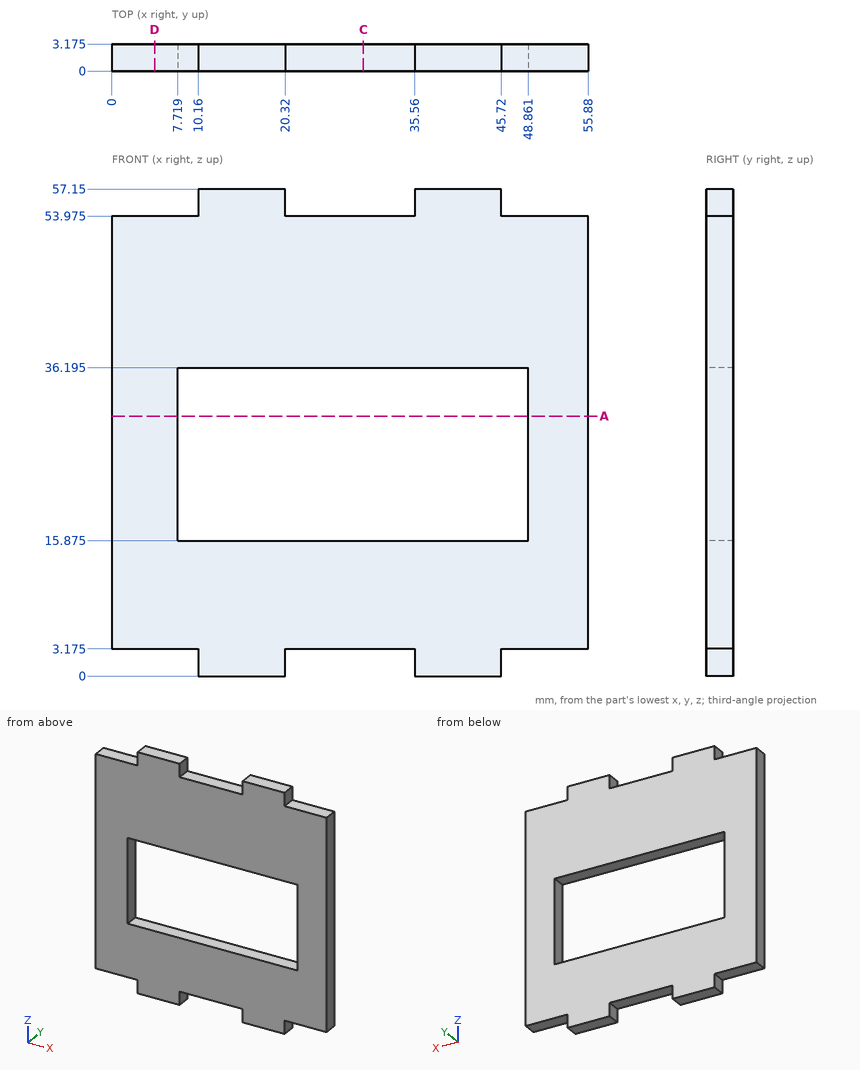
Drawing for the job (mm, zero at the part's lowest x, y, z). Round coordinates to 2 decimals unless told otherwise and drop trailing zeros. Order: outer loops, then holes, each group sorted by start corner. A loop starts at its lowest first (then second) coordinate and runs counter-clockwise, first axis right, second up.
Item 1: Saw through at C-C on x = 29.5. Write the cut outline in (y, z) (1 decimal).
Item 2: Saw through at A-A on z = 30.5. Write the cut outline in (x, y) (1 decimal), then the cut area to 3 significant figures.
Item 3: Saw through at D-D on x = 5. Write the cut outline in (y, z) (1 decimal), then the cut area to 3 significant figures.
Item 4: Pin check, flat tips, straight feed: pin 1 (1.6 mm diameter, centred on x = 5, y = 1.5, fed in from +Z) (3 decimals); pin 2 (1.6 mm diameter, centred on y = 1, z = 2, fed in from +X); pin 3 (1.6 mm diameter, centred on y = 1.5, z = 1, fed in from -X). Stop position of each tip, or through.
Item 5: Probe line 1 along X through (y, z) = (2.8, 33); line 2 along Z through (x, y) = (29.5, 1.95) (1 decimal); line 3 along Z through (x, y) = (5.5, 2.35) (1 decimal). List the from-to ranges inside material, lowest first.
Reported:
1. outline: (0, 3.2) - (3.2, 3.2) - (3.2, 15.9) - (0, 15.9) - close; (0, 36.2) - (3.2, 36.2) - (3.2, 54) - (0, 54) - close
2. outline: (0, 0) - (7.7, 0) - (7.7, 3.2) - (0, 3.2) - close; (48.9, 0) - (55.9, 0) - (55.9, 3.2) - (48.9, 3.2) - close
2. area: 46.8 mm2
3. outline: (0, 3.2) - (3.2, 3.2) - (3.2, 54) - (0, 54) - close
3. area: 161 mm2
4. pin 1: stops at z = 53.975
4. pin 2: stops at x = 45.72
4. pin 3: stops at x = 10.16
5. line 1: x = 0 to 7.72, 48.86 to 55.88
5. line 2: z = 3.2 to 15.9, 36.2 to 54
5. line 3: z = 3.2 to 54
